from build123d import *

# Parameters (mm, degrees)
SKETCH2_R                   = 12
BOSS_EXTRUDE1_DEPTH         = 20
FILLET1_R                   = 6
TAP_DRILL_FOR_M4_TAP1_D     = 3.3
TAP_DRILL_FOR_M4_TAP1_DEPTH = 13
TAP_DRILL_FOR_M4_TAP1_TIP   = 0.991420021
CUT_EXTRUDE4_DEPTH          = 9
FILLET2_R                   = 6
SKETCH8_R                   = 16
CUT_EXTRUDE5_DEPTH          = 8
TAP_DRILL_FOR_M8_TAP1_D     = 6.8
CUT_EXTRUDE6_DEPTH          = 2
SKETCH13_R                  = 7
CUT_EXTRUDE7_DEPTH          = 4
CHAMFER1_SIZE               = 0.5
CHAMFER2_SIZE               = 0.5


with BuildPart() as part:
    # Sketch2 → Boss-Extrude1 (new body)
    with BuildSketch(Plane(origin=(0, 0, 0), x_dir=(1, 0, 0), z_dir=(0, 1, 0))):
        with BuildLine():
            Line((-57, 40), (62, 40))
            Line((62, 40), (62, 55))
            ThreePointArc((62, 55), (76, 69), (90, 55))
            Line((90, 55), (90, -40))
            Line((90, -40), (-22, -40))
            Line((-22, -40), (-57, -5))
            Line((-57, -5), (-57, 40))
        make_face()
        with Locations((-35, 18.5)):
            Circle(SKETCH2_R, mode=Mode.SUBTRACT)
    extrude(amount=BOSS_EXTRUDE1_DEPTH)

    # Fillet1
    fillet1_edges = [part.edges().sort_by_distance(p)[0] for p in [
        (90, 10, 40),
        (-22, 10, 40),
        (-57, 10, 5),
        (-57, 10, -40),
        (62, 10, -40),
    ]]
    fillet(fillet1_edges, radius=FILLET1_R)

    # Tap Drill for M4 Tap1
    with Locations(Plane(origin=(0, 20, 0), x_dir=(1, 0, 0), z_dir=(0, 1, 0))):
        with Locations((-19.514718626, -34), (-52.5, 34), (84, -34), (84, 34)):
            Hole(TAP_DRILL_FOR_M4_TAP1_D / 2, depth=TAP_DRILL_FOR_M4_TAP1_DEPTH)
            with Locations((0, 0, -(TAP_DRILL_FOR_M4_TAP1_DEPTH + TAP_DRILL_FOR_M4_TAP1_TIP / 2))):  # 118° drill point
                Cone(0, TAP_DRILL_FOR_M4_TAP1_D / 2, TAP_DRILL_FOR_M4_TAP1_TIP, mode=Mode.SUBTRACT)

    # Sketch7 → Cut-Extrude4 (cut)
    with BuildSketch(Plane(origin=(0, 20, 0), x_dir=(1, 0, 0), z_dir=(0, 1, 0))):
        with BuildLine():
            Line((-52.5, 18.5), (-52.5, -1.357864376))
            ThreePointArc((-52.5, -1.357864376), (-52.043277195, -3.65396497), (-50.742640687, -5.600505063))
            Line((-50.742640687, -5.600505063), (-25.115965744, -31.227180006))
            ThreePointArc((-25.115965744, -31.227180006), (-17.122947173, -28.225752922), (-13.593358985, -36))
            Line((-13.593358985, -36), (78.078640359, -36))
            ThreePointArc((78.078640359, -36), (79.580582618, -29.580582618), (86, -28.078640359))
            Line((86, -28.078640359), (86, 28.078640359))
            ThreePointArc((86, 28.078640359), (79.580582618, 29.580582618), (78.078640359, 36))
            Line((78.078640359, 36), (-35, 36))
            ThreePointArc((-35, 36), (-47.374368671, 30.874368671), (-52.5, 18.5))
        make_face()
    extrude(amount=-CUT_EXTRUDE4_DEPTH, mode=Mode.SUBTRACT)

    # Fillet2
    fillet2_edges = [part.edges().sort_by_distance(p)[0] for p in [
        (86, 15.5, 28.078640359),
        (78.078640359, 15.5, 36),
        (-13.593358985, 15.5, 36),
        (-25.115965744, 15.5, 31.227180006),
        (78.078640359, 15.5, -36),
        (86, 15.5, -28.078640359),
    ]]
    fillet(fillet2_edges, radius=FILLET2_R)

    # Sketch8 → Cut-Extrude5 (cut)
    with BuildSketch(Plane(origin=(0, 11, 0), x_dir=(1, 0, 0), z_dir=(0, 1, 0))):
        with Locations((-35, 18.5)):
            Circle(SKETCH8_R)
    extrude(amount=-CUT_EXTRUDE5_DEPTH, mode=Mode.SUBTRACT)

    # Tap Drill for M8 Tap1 (through all)
    with Locations(Plane(origin=(0, 20, 0), x_dir=(1, 0, 0), z_dir=(0, 1, 0))):
        with Locations((76, 55)):
            Hole(TAP_DRILL_FOR_M8_TAP1_D / 2)

    # Sketch12 → Cut-Extrude6 (cut)
    with BuildSketch(Plane(origin=(0, 20, 0), x_dir=(1, 0, 0), z_dir=(0, 1, 0))):
        with BuildLine():
            Line((84, 40), (50.858800106, 40))
            Line((50.858800106, 40), (50.858800106, 55))
            ThreePointArc((50.858800106, 55), (76, 80.141199894), (101.141199894, 55))
            Line((101.141199894, 55), (101.141199894, 34))
            Line((101.141199894, 34), (90, 34))
            ThreePointArc((90, 34), (88.242640687, 38.242640687), (84, 40))
        make_face()
    extrude(amount=-CUT_EXTRUDE6_DEPTH, mode=Mode.SUBTRACT)

    # Sketch13 → Cut-Extrude7 (cut)
    with BuildSketch(Plane(origin=(0, 18, 0), x_dir=(1, 0, 0), z_dir=(0, 1, 0))):
        with Locations((76, 55)):
            Circle(SKETCH13_R)
    extrude(amount=-CUT_EXTRUDE7_DEPTH, mode=Mode.SUBTRACT)

    # Chamfer1
    chamfer1_edges = [part.edges().sort_by_distance(p)[0] for p in [
        (62, 0, -50.5),
        (76, 0, -69),
        (90, 0, -10.5),
        (-47, 0, -18.5),
        (79.4, 0, -55),
        (32.242640687, 0, 40),
        (-39.5, 0, 22.5),
        (-57, 0, -15.742640687),
        (2.5, 0, -40),
        (88.242640687, 0, 38.242640687),
        (-55.242640687, 0, -38.242640687),
        (-56.543277195, 0, 4.81081922),
        (-21.81081922, 0, 39.543277195),
        (60.242640687, 0, -41.757359313),
    ]]
    chamfer(chamfer1_edges, length=CHAMFER1_SIZE)

    # Chamfer2
    chamfer2_edges = [part.edges().sort_by_distance(p)[0] for p in [
        (-17.122947173, 20, 28.225752922),
        (32.242640687, 20, 36),
        (79.580582618, 20, -29.580582618),
        (86, 20, 0),
        (18.710731912, 20, -36),
        (79.580582618, 20, 29.580582618),
        (-25.866850849, 20, 28.901520169),
        (-11.417913194, 20, 34.886466108),
        (84.886466108, 20, -25.903194568),
        (75.903194568, 20, -34.886466108),
        (84.886466108, 20, 25.903194568),
        (75.903194568, 20, 34.886466108),
        (-51, 11, -18.5),
        (69, 18, -55),
        (-47.374368671, 20, -30.874368671),
        (-52.5, 20, -8.571067812),
        (-52.043277195, 20, 3.65396497),
        (-39.929417161, 20, 16.413728589),
    ]]
    chamfer(chamfer2_edges, length=CHAMFER2_SIZE)


solid = part.part
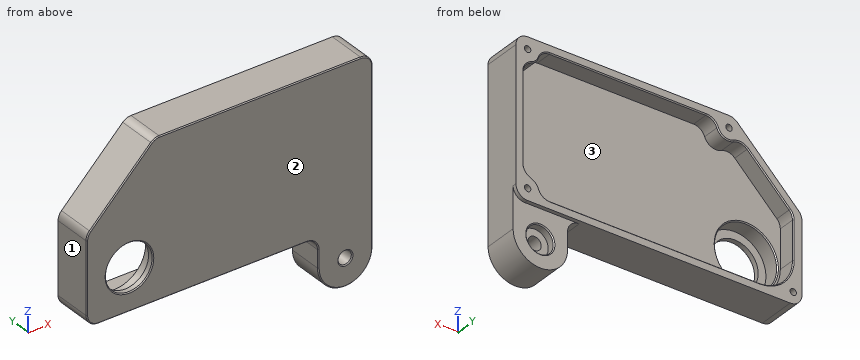
Check sheet for the modelled part. Datum: model origin and axes. Units: mm. Face numbers are marked on the shaded views. Give positions to 0.01 mm unless a question says otherwise; leave off trailing zeros. Write each loop counter-clockwise with the first axis right and the second up, starting at its lowest first coordinate (ties: lowest second). Pieces come first, ordered by that corner, then holes. Notation, with made-up numbers: (34, -22.75) -> (61, -22.75) arc R19 ccw to (61, -13.75) -> close; hole circle Ø11 at (22, -30). An arc over 180 degrees is marked (long way). Use one line per item in the form item = value. Start each with the question number.
1. Mould release check, pull along X, two halves, no side actions. Record for the marked faces 1, 2 and 3: pulls with the +X half, pulls with the -X half, needs draft (parallel to the pull), parting line crosses it, or undercut.
2. Go/stop test with flat-tipped pins: P1, Ø4, axis at y = 15.5, z = 10, coming from the -X side; P2, Ø9.5, axis at x = 25.5, y = 16.5, coming from the -Z side; P3, Ø2, axis at x = 65, y = 5, coming from the -Z side. Record where each tip stops, or that it passes through.
3. Thickness scan on line 1 along X through (y, z) = (14, 34); line 2 along Z through (x, y) = (76, 15.1); line 3 along Z through (x, y) = (19, 12). Record the ranges inside material, lowest first. Write a range as from..to.
4. Section check A-A (x = 2). Record the cut outline in (y, z).
5. Section check B-B (z = 18.5). Record the cut outline in (x, y), and give its area (3 significant figures).
Conclusion:
q1.face_1 = pulls with the -X half
q1.face_2 = needs draft
q1.face_3 = undercut
q2.P1 = -54
q2.P2 = -40
q2.P3 = -64.8
q3.line_1 = -28..-21.16, -17.86..-12.41, 76.89..82.35, 85.65..90
q3.line_2 = -69..-62, -48..-34.82, 34.82..40
q3.line_3 = -40..-36, 36..40
q4.outline = (0, -39.5) -> (0.5, -40) -> (20, -40) -> (20, -36.5) -> (19.5, -36) -> (11, -36) -> (11, 36) -> (19.5, 36) -> (20, 36.5) -> (20, 40) -> (0.5, 40) -> (0, 39.5) -> close
q5.outline = (-43.5, 0.5) -> (-42.79, 0) -> (89.5, 0) -> (90, 0.5) -> (90, 20) -> (86.5, 20) -> (86, 19.5) -> (86, 11) -> (-37.84, 11) -> (-37.84, 19.5) -> (-38.55, 20) -> (-43.5, 20) -> close
q5.area = 1,550 mm²
